Verification items for this drawing (mm, ordinates from the low corner). A direction names the side the tool comes from. Round coordinates to 2 decimals unless told otherwise and drop trailing zeros. Loops run counter-clockwise (first coordinate to the right, second up) from the corner with the lowest first, then second, coordinate; pieces in that order, holes last. Notation, with made-up numbers: M 77,-34 L 117,-34 A24 cw 117,-10 Z; hole C 56,34.5 d11. An arc over 180 degrees is marked long. Answer as CSV lines item,"result".
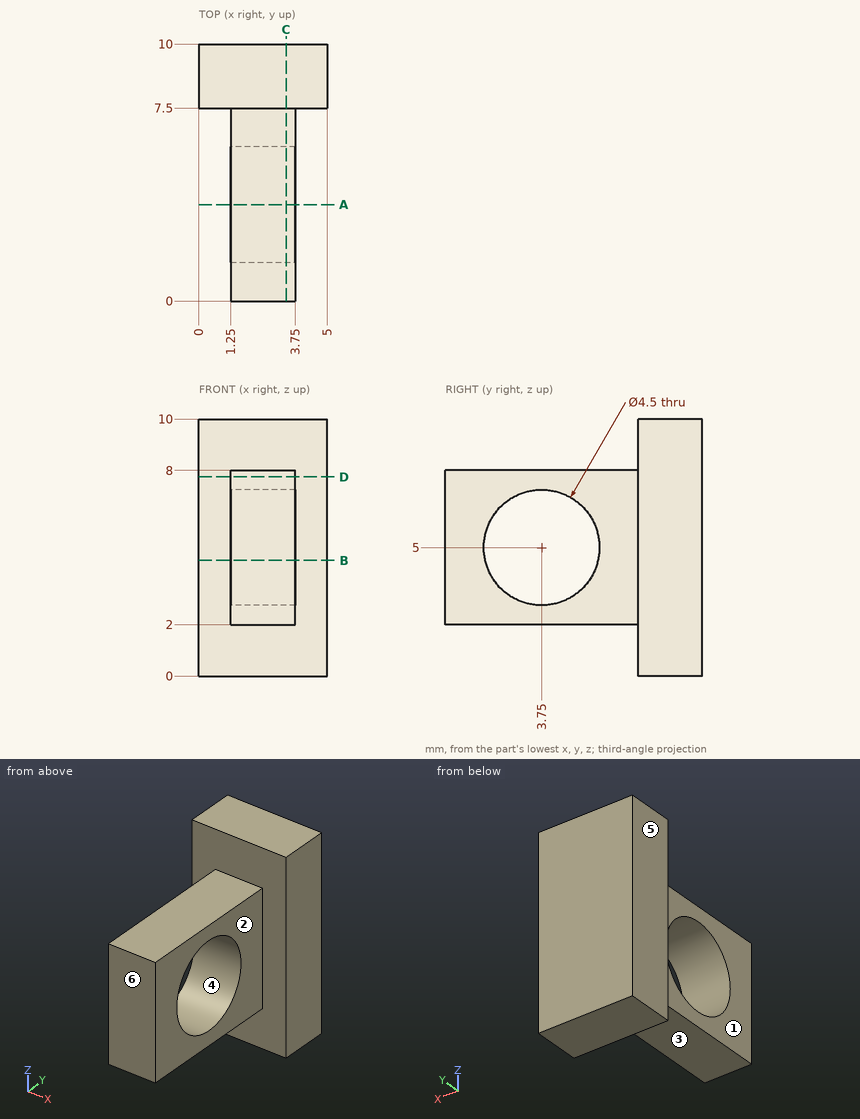
1) Section check C-C (x = 3.4). Record the cut outline in (y, z).
Here are the results:
outline,"M 0,2 L 7.5,2 L 7.5,0 L 10,0 L 10,10 L 7.5,10 L 7.5,8 L 0,8 Z; hole C 3.75,5 d4.5"
2) Set-up check for the marked faces 1, 2 and 3: record each of +Z, -Z, +X, -X, +Y, -Y from which the full face is reachable in a straight line by a thin tool's end or side.
Here are the results:
face 1,"+Z, -Z, -X, -Y"
face 2,"+Z, -Z, +X, -Y"
face 3,"-Z, +X, -X, -Y"
3) Material ranges on probe 1 along Z at (x, y) = (2.65, 3.75); probe 2 along Y at (x, z) = (2.7, 1.25); probe 3 along X at (y, z) = (1.25, 5.75), recorded low to high.
Here are the results:
probe 1,"z = 2 to 2.75, 7.25 to 8"
probe 2,"y = 7.5 to 10"
probe 3,"x = 1.25 to 3.75"
4) Draft check along Y on the marked faces 4, 5 and 6. Enter one of: +Y half, -Y half, draft (parallel to the pull), parting line (faces both ways), or undercut.
Here are the results:
face 4,"undercut"
face 5,"draft"
face 6,"-Y half"
5) Section check A-A (y = 3.75). Record the cut outline in (x, z), plus the area to 3 significant figures.
Here are the results:
outline,"M 1.25,2 L 3.75,2 L 3.75,2.75 L 1.25,2.75 Z; M 1.25,7.25 L 3.75,7.25 L 3.75,8 L 1.25,8 Z"
area,"3.75 mm^2"
6) Go/stop test with flat-tipped pins: pin 1 (4 mm diameter, centred on y = 4.5, z = 6.5, fed in from -X); pin 2 (0.8 mm diameter, centred on x = 2, y = 5, fed in from +Z); pin 3 (0.8 mm diameter, centred on x = 2.5, y = 2.5, fed in from -Z). Record where each tip stops, or that it passes through.
Here are the results:
pin 1,"stops at x = 1.25"
pin 2,"stops at z = 8"
pin 3,"stops at z = 2"
7) Section check B-B (z = 4.5). Record the cut outline in (x, y).
Here are the results:
outline,"M 0,7.5 L 1.25,7.5 L 1.25,5.94 L 3.75,5.94 L 3.75,7.5 L 5,7.5 L 5,10 L 0,10 Z; M 1.25,0 L 3.75,0 L 3.75,1.56 L 1.25,1.56 Z"
8) Section check D-D (z = 7.75). Record the cut outline in (x, y), plus the area to 4 significant figures.
Here are the results:
outline,"M 0,7.5 L 1.25,7.5 L 1.25,0 L 3.75,0 L 3.75,7.5 L 5,7.5 L 5,10 L 0,10 Z"
area,"31.25 mm^2"
